Verification items for the finished model (mm, model axes). A direction names the side the tool comes from. Round coordinates to 2 decimals unless told otherwise and drop trailing zeros. Write each loop counter-clockwise with the first axis right and the second up, starting at its lowest first coordinate (ties: lowest second). Pieces come first, ordered by that corner, then holes.
from build123d import *

# Parameters (mm, degrees)
SKETCH3_W                      = 21.924187445
SKETCH3_H                      = 19.837641971
BOSS_EXTRUDE1_DEPTH            = 6.35
SKETCH4_R                      = 3.175
CUT_EXTRUDE1_DEPTH             = 9.525
SKETCH5_R                      = 3.175
CUT_EXTRUDE5_DEPTH             = 9.525
CUT_EXTRUDE5_DIRECTION_2_REACH = 27.174
SKETCH6_R                      = 3.175
CUT_EXTRUDE6_DEPTH             = 9.525
SKETCH7_W                      = 12.7
SKETCH7_H                      = 1.803641971
CUT_EXTRUDE7_DEPTH             = 31.241106695


with BuildPart() as part:
    # Sketch3 → Boss-Extrude1 (new, symmetric)
    with BuildSketch(Plane.XY):
        with Locations((10.962093723, -9.918820986)):
            Rectangle(SKETCH3_W, SKETCH3_H)
    extrude(amount=BOSS_EXTRUDE1_DEPTH, both=True)

    # Sketch4 → Cut-Extrude1 (cut)
    with BuildSketch(Plane.ZY):
        with Locations(Location((0, -6.35, 0), (0, 0, 270))):
            Circle(SKETCH4_R)
    extrude(amount=-CUT_EXTRUDE1_DEPTH, mode=Mode.SUBTRACT)

    # Sketch5 → Cut-Extrude5 (cut)
    with BuildSketch(Plane(origin=(7.787093723, -19.837641971, 0), x_dir=(-0.8660254037844382, 0.500000000000001, 0), z_dir=(-0.500000000000001, -0.8660254037844382, 0))):
        with Locations(Location((0, 0, 0), (0, 0, 180))):
            Circle(SKETCH5_R)
    extrude(amount=-CUT_EXTRUDE5_DEPTH, mode=Mode.SUBTRACT)

    # Sketch5 → Cut-Extrude5 direction 2 (cut, up to next)
    with BuildSketch(Plane(origin=(7.787093723, -19.837641971, 0), x_dir=(-0.8660254037844382, 0.500000000000001, 0), z_dir=(-0.500000000000001, -0.8660254037844382, 0)), mode=Mode.PRIVATE) as cut_extrude5_direction_2_sk1:
        with Locations(Location((0, 0, 0), (0, 0, 180))):
            Circle(SKETCH5_R)
    cut_extrude5_direction_2_tool1 = extrude(cut_extrude5_direction_2_sk1.sketch, amount=CUT_EXTRUDE5_DIRECTION_2_REACH, mode=Mode.PRIVATE) & part.part
    add(cut_extrude5_direction_2_tool1.solids().sort_by_distance((7.787094, -19.837642, 0))[0], mode=Mode.SUBTRACT)

    # Sketch6 → Cut-Extrude6 (cut)
    with BuildSketch(Plane(origin=(0, 0, -6.35), x_dir=(-1, 0, 0), z_dir=(0, 0, -1))):
        with Locations((-15.574187445, -6.35)):
            Circle(SKETCH6_R)
    extrude(amount=-CUT_EXTRUDE6_DEPTH, mode=Mode.SUBTRACT)

    # Sketch7 → Cut-Extrude7 (cut, through all)
    with BuildSketch(Plane(origin=(21.924187445, 0, 0), x_dir=(0, 0, -1), z_dir=(1, 0, 0))):
        with Locations((0, -18.935820986)):
            Rectangle(SKETCH7_W, SKETCH7_H)
    extrude(amount=-CUT_EXTRUDE7_DEPTH, mode=Mode.SUBTRACT)


solid = part.part
Q1. Sectioned sample at C-C (x = 18.25). Enter the section's corners in (y, z) (3 decimals), plus the area to 3 significant figures.
Recorded:
outline: (-18.034, -6.35) - (-8.059, -6.35) - (-8.059, 3.175) - (-4.641, 3.175) - (-4.641, -6.35) - (0, -6.35) - (0, 6.35) - (-18.034, 6.35) - close
area: 196 mm2
Q2. Depth check by flat-ended pin: P1, Ø5.5, axis at y = -6.35, z = 0, coming from the -X side (3 decimals); P2, Ø3, axis at x = 16, y = -6, coming from the -Z side (3 decimals); P3, Ø1.5, axis at x = 8, z = -1, coming from the -Y side. Enter the tip coordinate at first touch or a pass-through.
Recorded:
P1: stops at x = 9.525
P2: stops at z = 3.175
P3: stops at y = -14.87
Q3. Material ranges on line 1 along Z through (x, y) = (4.5, -6.35) (3 decimals); line 2 along Y through (x, z) = (7, 1); line 3 along X through (y, z) = (-8.5, 2.5), recorded low to high.
Recorded:
line 1: z = -6.35 to -3.175, 3.175 to 6.35
line 2: y = -15.17 to -9.36, -3.34 to 0
line 3: x = 0 to 13.24, 17.91 to 21.92
Q4. Tool access check on faces 1 (the cylindrical face through (4.7, -3.18, 0.14)), 2 (the flat face through (12.511, -11.567, 0.044)), 3 (the flat face through (11, -9, -6.35)), 4 (the flat face through (16, -6, 3.175)), 5 (the flat face through (0, -11, 0)). Record the directions out of +Z, -Z, +X, -X, +Y, -Y that give a thin tool (end or side, any length) a straight path to the whole face; none if there is none.
Recorded:
face 1: -X
face 2: none
face 3: -Z, +X, -X, +Y, -Y
face 4: -Z
face 5: +Z, -Z, -X, +Y, -Y
Q5. Sectioned sample at A-A (y = -6.35). Enter the section's corners in (x, z) (3 decimals), plus the area to 3 significant figures.
Recorded:
outline: (0, -6.35) - (12.399, -6.35) - (12.399, 3.175) - (18.749, 3.175) - (18.749, -6.35) - (21.924, -6.35) - (21.924, 6.35) - (0, 6.35) - (0, 3.175) - (9.525, 3.175) - (9.525, -3.175) - (0, -3.175) - close
area: 157 mm2
Q6. Release check for a two-part mould opening along Y. For faces 6 (the flat face through (21.924, -9, 0)), 7 (the flat face through (11, 0, 0)), 8 (the cylindrical face through (16.26, -9.45, -1.65)), 9 (the flat face through (14, -18.034, 0)) record: released by +Y, released by -Y, zero draft, split by the parting line, or undercut.
Recorded:
face 6: zero draft
face 7: released by +Y
face 8: undercut
face 9: released by -Y
